Build history of the part. All positions in model axes, mm. Round coordinates to 2 decimals unless told otherwise and drop trailing zeros. Write each loop counter-clockwise with the first axis right and the second up, starting at its lowest first coordinate (ties: lowest second). Pieces come first, ordered by that corner, then holes.
1) Saw through at A-A (x = 0). Write the cut outline in (y, z), plus the area to 3 significant figures.
2) Wall check: probe 1 along Y at (x, z) = (0, 5.25); probe 2 along Y at (x, z) = (0, 2.3). Give the ranges that are in metal, low to high.
3) Saw through at B-B (y = 0). Write the cut outline in (x, z).
4) Flat gauge pins, fed straight in: pin 1 (5 mm diameter, centred on x = 0, y = 0, fed in from -Z); pin 2 (8 mm diameter, centred on x = 0, y = 0, fed in from -Z). Where does each tip first touch, or does it go through?
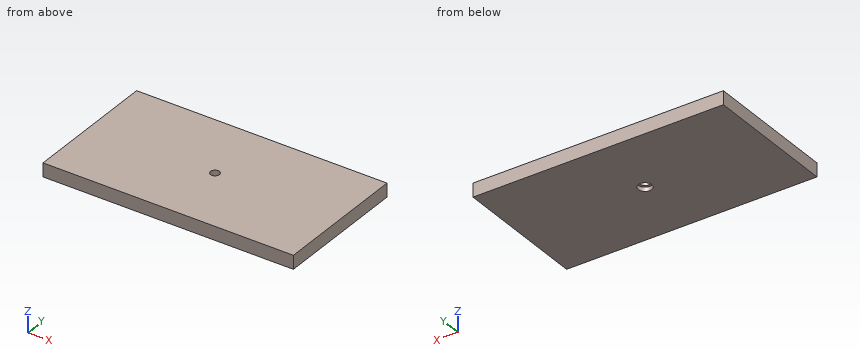
from build123d import *

# Parameters (mm, degrees)
F0_W     = 183.6964
F0_H     = 99.261144
F0_R     = 3.25
F1_DEPTH = 10
F2_R     = 3.25
F3_DEPTH = 3


with BuildPart() as f1:
    # F0 (on Top) → F1 (new body)
    with BuildSketch(Plane.XY):
        Rectangle(F0_W, F0_H)
        Circle(F0_R, mode=Mode.SUBTRACT)
    extrude(amount=F1_DEPTH)

    # F2 (on face) → F3 (cut)
    with BuildSketch(Plane.XY):
        with BuildLine():
            ThreePointArc((-5, 0), (0, -5), (5, 0))
            ThreePointArc((5, 0), (0, 5), (-5, 0))
        make_face()
        Circle(F2_R, mode=Mode.SUBTRACT)
    extrude(amount=F3_DEPTH, mode=Mode.SUBTRACT)


solid = f1.part
Evaluation:
1. outline: (-49.63, 0) - (-5, 0) - (-5, 3) - (-3.25, 3) - (-3.25, 10) - (-49.63, 10) - close; (3.25, 3) - (5, 3) - (5, 0) - (49.63, 0) - (49.63, 10) - (3.25, 10) - close
1. area: 917 mm2
2. probe 1: y = -49.63 to -3.25, 3.25 to 49.63
2. probe 2: y = -49.63 to -5, 5 to 49.63
3. outline: (-91.85, 0) - (-5, 0) - (-5, 3) - (-3.25, 3) - (-3.25, 10) - (-91.85, 10) - close; (3.25, 3) - (5, 3) - (5, 0) - (91.85, 0) - (91.85, 10) - (3.25, 10) - close
4. pin 1: passes through
4. pin 2: stops at z = 3
